Model file for the job. Use its own axes, mm. Round coordinates to 2 decimals unless told otherwise and drop trailing zeros. Loops run counter-clockwise (first coordinate to the right, second up) from the corner with the lowest first, then second, coordinate; pieces in that order, holes last. Notation, with made-up numbers: M 5,29 L 30,29 A13 cw 30,37 Z; hole C 5.25,54 d9. An arc over 180 degrees is marked long. Use a Markdown table: item, result. Add a question column.
Item 1: Pin check, flat tip, straight feed: P1, Ø2.5, axis at x = 560.96, z = -127.86, coming from the +Y side. Stop position of the tip, or through.
Item 2: Saw through at C-C on y = 1.5. Give the number of separate pieces and of enclosed holes in the cut face, then the cut area to 3 significant figures.
Item 3: Wall check: L1, parallel to X at y = 4, z = -63.5; L2, parallel to Z at x = -51, y = 4.5; L3, parallel to X at y = 4, z = 16. Give the ranges that are in metal, low to high. Write a range as from..to.
Item 4: Saw through at B-B on z = 36.5. Write the cut outline in (x, y), then the cut area to 3 significant figures.
Item 5: Two-plate mould, pull along Z, no slides. Class faces 1 (the flat face through (223, 6.35, -48)), 2 (the cylindrical face through (427.22, 3.22, -60.76)): +Z half, -Z half, draft (parallel to the pull), parting line (faces both ways), or undercut.
Item 6: Saw through at A-A on z = -63.5. Write the cut outline in (x, y), then the cut area to 3 significant figures.
Item 7: Saw through at D-D on x = 237. Write the cut outline in (y, z), then the cut area to 3 significant figures.
```python
from build123d import *

# Parameters (mm, degrees)
BOSS_EXTRUDE1_DEPTH = 6.35
SKETCH3_R           = 3.175
SKETCH3_R_2         = 1.905
SKETCH3_R_3         = 7.14375
CUT_EXTRUDE1_DEPTH  = 7.62


with BuildPart() as part:
    # Sketch1 → Boss-Extrude1 (new body)
    with BuildSketch(Plane(origin=(0, 0, 0), x_dir=(1, 0, 0), z_dir=(0, 1, 0))):
        Polygon((0, 0), (457.2, 0), (457.2, -50.8), (609.6, -50.8), (609.6, 144.78), (-152.4, 144.78), (-152.4, -50.8), (0, -50.8), align=None)
    extrude(amount=BOSS_EXTRUDE1_DEPTH)

    # Sketch3 → Cut-Extrude1 (cut)
    with BuildSketch(Plane(origin=(0, 6.35, 0), x_dir=(1, 0, 0), z_dir=(0, 1, 0))):
        with Locations((-139.7, -25.4)):
            Circle(SKETCH3_R)
        with Locations((-99.1108, 84.8106)):
            Circle(SKETCH3_R_2)
        with Locations((-142.875, 126.81712)):
            Circle(SKETCH3_R)
        with Locations((-51.435, 84.8106)):
            Circle(SKETCH3_R_2)
        with Locations((-51.435, 127.8636)):
            Circle(SKETCH3_R_2)
        with Locations((36.576, 63.5)):
            Circle(SKETCH3_R_3)
        with Locations((600.075, 126.81712)):
            Circle(SKETCH3_R)
        with Locations((596.9, -25.4)):
            Circle(SKETCH3_R)
        with Locations((560.959, 127.8636)):
            Circle(SKETCH3_R_2)
        with Locations((513.207, 84.8106)):
            Circle(SKETCH3_R_2)
        with Locations((560.959, 84.8106)):
            Circle(SKETCH3_R_2)
        with Locations((513.207, 126.81712)):
            Circle(SKETCH3_R_2)
        with Locations((420.624, 63.5)):
            Circle(SKETCH3_R_3)
        with Locations((-99.1108, 127.8636)):
            Circle(SKETCH3_R_2)
    extrude(amount=-CUT_EXTRUDE1_DEPTH, mode=Mode.SUBTRACT)


solid = part.part
```
Entries:
| question | item | result |
|---|---|---|
| 1 | P1 | through |
| 2 | separate pieces | 1 |
| 2 | enclosed holes | 14 |
| 2 | area | 125,000 mm2 |
| 3 | L1 | -152.4..29.43, 43.72..413.48, 427.77..609.6 |
| 3 | L2 | -144.78..-129.72, -126.01..-86.67, -82.96..50.8 |
| 3 | L3 | -152.4..0, 457.2..609.6 |
| 4 | outline | M -152.4,0 L 0,0 L 0,6.35 L -152.4,6.35 Z; M 457.2,0 L 609.6,0 L 609.6,6.35 L 457.2,6.35 Z |
| 4 | area | 1,940 mm2 |
| 5 | face 1 | draft |
| 5 | face 2 | undercut |
| 6 | outline | M -152.4,0 L 29.43,0 L 29.43,6.35 L -152.4,6.35 Z; M 43.72,0 L 413.48,0 L 413.48,6.35 L 43.72,6.35 Z; M 427.77,0 L 609.6,0 L 609.6,6.35 L 427.77,6.35 Z |
| 6 | area | 4,660 mm2 |
| 7 | outline | M 0,-144.78 L 6.35,-144.78 L 6.35,0 L 0,0 Z |
| 7 | area | 919 mm2 |
